from build123d import *
from build123d.topology import SkipClean

# Parameters (mm, degrees)
BOSS_EXTRUDE2_DEPTH = 60.96
SKETCH2_R           = 71.12
BOSS_EXTRUDE3_DEPTH = 81.28
CUT_EXTRUDE1_DEPTH  = 101.6
CUT_EXTRUDE2_START  = -142.24
CUT_EXTRUDE2_DEPTH  = 142.24


with BuildPart() as part:
    # Sketch1 → Boss-Extrude2 (new body)
    with BuildSketch(Plane(origin=(0, 0, 0), x_dir=(1, 0, 0), z_dir=(0, 1, 0))):
        with BuildLine():
            Line((228.6, 60.96), (228.6, -60.96))
            Line((228.6, -60.96), (36.632400959, -60.96))
            ThreePointArc((36.632400959, -60.96), (-71.12, 0), (36.632400959, 60.96))
            Line((36.632400959, 60.96), (228.6, 60.96))
        make_face()
    extrude(amount=BOSS_EXTRUDE2_DEPTH)

    # Sketch2 → Boss-Extrude3 (add)
    with SkipClean():  # the faces are left unmerged after this step: merging them gives an invalid solid
        with BuildSketch(Plane(origin=(0, 60.96, 0), x_dir=(1, 0, 0), z_dir=(0, 1, 0))):
            with Locations(Location((0, 0, 0), (0, 0, 58.997280866))):
                Circle(SKETCH2_R)
        extrude(amount=BOSS_EXTRUDE3_DEPTH)

    # Sketch3 → Cut-Extrude1 (cut)
    with SkipClean():  # the faces are left unmerged after this step: merging them gives an invalid solid
        with BuildSketch(Plane(origin=(228.6, 0, 0), x_dir=(0, 0, -1), z_dir=(1, 0, 0))):
            with BuildLine():
                Line((40.64, 60.96), (-40.64, 60.96))
                ThreePointArc((-40.64, 60.96), (0, 20.32), (40.64, 60.96))
            make_face()
        extrude(amount=-CUT_EXTRUDE1_DEPTH, mode=Mode.SUBTRACT)

    # Sketch4 → Cut-Extrude2 (cut)
    with SkipClean():  # the faces are left unmerged after this step: merging them gives an invalid solid
        with BuildSketch(Plane(origin=(0, 142.24, 0), x_dir=(1, 0, 0), z_dir=(0, 1, 0)).offset(CUT_EXTRUDE2_START)):
            with BuildLine():
                Line((-39.91923346, 7.62), (-70.710607408, 7.62))
                ThreePointArc((-70.710607408, 7.62), (-71.12, 0), (-70.710607408, -7.62))
                Line((-70.710607408, -7.62), (-39.91923346, -7.62))
                ThreePointArc((-39.91923346, -7.62), (40.64, 0), (-39.91923346, 7.62))
            make_face()
        extrude(amount=CUT_EXTRUDE2_DEPTH, mode=Mode.SUBTRACT)


solid = part.part
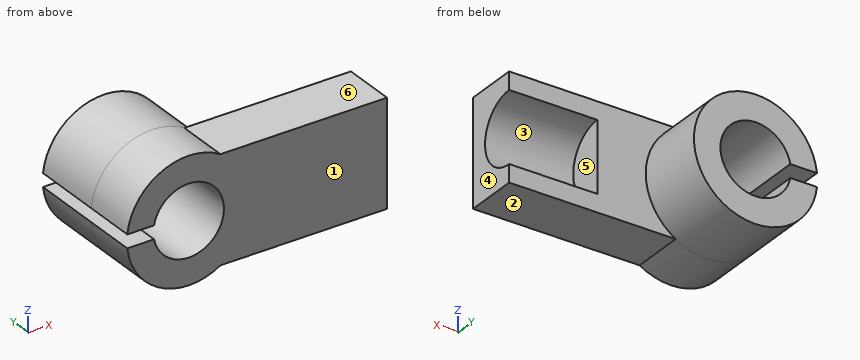
Geometry check sheet. Reference: the model listing, model coordinates, mm. Face numbers are marked on the shaded views. A direction names the side the tool comes from. Round coordinates to 2 decimals unless told otherwise and drop trailing zeros. Write each loop counter-clockwise with the first axis right and the second up, starting at its lowest first coordinate (ties: lowest second). Pieces come first, ordered by that corner, then holes. Notation, with made-up numbers: (29.25, -34.5) - (72.25, -34.5) arc R20 ccw to (72.25, -28.5) - close; hole circle Ø3 at (71.5, 53). An arc over 180 degrees is marked (long way). One line per item, written item: value.
1. Depth check by flat-ended pin: pin 1 Ø8 at (x, y) = (-14, 69) entering from -Z; pin 2 Ø15.5 at (x, y) = (-50, 42) entering from -Z; pin 3 Ø4 at (y, z) = (73.5, -34) entering from +X. Enter the tip coordinate at first touch or a pass-through.
The answers:
pin 1: stops at z = -70.41
pin 2: stops at z = -57.21
pin 3: stops at x = 63.51
2. Mould release check, pull along Z, two halves, no side actions. Record for the marked faces 4, 5 and 6: released by +Z, released by -Z, zero draft, split by the parting line, or undercut.
The answers:
face 4: zero draft
face 5: undercut
face 6: released by +Z
3. Cross-section at D-D on z = 0. Record the boundary of the cut face in (x, y).
The answers:
outline: (40.64, 0) - (228.6, 0) - (228.6, 20.32) - (127, 20.32) - (127, 60.96) - (71.12, 60.96) - (71.12, 142.24) - (40.64, 142.24) - close
4. Scan lines: L1, parallel to Z at x = 0, y = 64; L2, parallel to Y at x = 114, z = -25.5; L3, parallel to Z at x = 92, y = 46. Record each from-to range of solid material in increasing order.
The answers:
L1: z = -71.12 to -40.64, 40.64 to 71.12
L2: y = 0 to 60.96
L3: z = -60.96 to 60.96
5. Set-up check for the marked faces 1, 2 and 3: record each of +Z, -Z, +X, -X, +Y, -Y from which the full face is reachable in a straight line by a thin tool's end or side.
The answers:
face 1: +Z, -Z, +X, -X, -Y
face 2: -Z, +X, +Y, -Y
face 3: +X, +Y
6. Cross-section at B-B on z = 29.5. Record the boundary of the cut face in (x, y).
The answers:
outline: (-64.71, 0) - (-27.95, 0) - (-27.95, 142.24) - (-64.71, 142.24) - close; (27.95, 0) - (228.6, 0) - (228.6, 33.01) - (127, 33.01) - (127, 60.96) - (64.71, 60.96) - (64.71, 142.24) - (27.95, 142.24) - close
7. Cross-section at A-A on x = 0. Record the boundary of the cut face in (y, z).
The answers:
outline: (0, -71.12) - (142.24, -71.12) - (142.24, -40.64) - (0, -40.64) - close; (0, 40.64) - (142.24, 40.64) - (142.24, 71.12) - (0, 71.12) - close
8. Cross-section at C-C on y = 12. Record the boundary of the cut face in (x, z).
The answers:
outline: (-70.71, -7.62) arc R71.12 ccw to (36.63, -60.96) - (228.6, -60.96) - (228.6, 60.96) - (36.63, 60.96) arc R71.12 ccw to (-70.71, 7.62) - (-39.92, 7.62) arc R40.64 cw (long way) to (-39.92, -7.62) - close
